Autodesk Inventor part; units mm, degrees
ref_plane "YZ Plane" through (0, 0, 0) normal (1, 0, 0) x (0, 1, 0)
ref_plane "XZ Plane" through (0, 0, 0) normal (0, 1, 0) x (-1, 0, 0)
ref_plane "XY Plane" through (0, 0, 0) normal (0, 0, 1) x (1, 0, 0)
sketch "Sketch1" plane through (0, 0, 0) normal (0, 0, 1) x (1, 0, 0)
  line L0 (-568.325, -1219.2) -> (568.325, -1219.2)
  line L1 (568.325, -1219.2) -> (568.325, 1219.2)
  line L2 (568.325, 1219.2) -> (-568.325, 1219.2)
  line L3 (-568.325, 1219.2) -> (-568.325, -1219.2)
  line L4 (-568.325, -1219.2) -> (568.325, 1219.2) construction
  line L5 (568.325, -1219.2) -> (-568.325, 1219.2) construction
  line L6 (568.325, 1219.2) -> (-568.325, -1219.2)
  line L7 (-528.0371, -1237.98) -> (-608.6129, -1200.42)
  line L8 (608.6129, 1200.42) -> (528.0371, 1237.98)
  line L9 (528.0371, 1237.98) -> (-608.6129, -1200.42)
  line L10 (-528.0371, -1237.98) -> (608.6129, 1200.42)
  point P0 (0, 0)
  point P1 (519.2829, 1219.2)
  point P2 (-568.325, -1113.9923)
  point P3 (-519.2829, -1219.2)
  point P4 (568.325, 1113.9923)
  dimension "d0" = 1136.65
  dimension "d1" = 2438.4
  dimension "d2" = 88.9
  dimension "d3" = 88.9
extrude "Extrusion1" add sketch "Sketch1" along normal blind 38.1 contours L6 L1 L10 L0 | L3 L9 L2 L6
properties part number "S_2x4x105.918"
Input: part model. Units: mm. Frame: model coordinates. Coordinates: 2 decimals unless noted, no trailing zeros. Order: outer loops, then holes, each group sorted by start corner. A loop starts at its lowest first (then second) coordinate and runs counter-clockwise, first axis right, second up. Notation, with made-up numbers: M 49.5,61.25 L 106.5,61.25 A24 ccw 106.5,88.25 Z; hole C 59,-19 d7. An arc over 180 degrees is marked long. Answer as CSV lines item,"result".
1. First-contact query: P1, Ø2, axis at x = 380, z = 18.5, coming from the +Y side; P2, Ø2, axis at x = 186, z = 31.5, coming from the -Y side; P3, Ø3, axis at x = 394.5, z = 20.5, coming from the -Y side. Flat tips, straight axial feed; report the tip coordinate or a pass-through.
Reported:
P1,"y = 922.55"
P2,"y = 291.66"
P3,"y = 737.88"
2. Section A-A (z = 6). Return the cut outline in (x, y) (3 decimals).
Reported:
outline,"M -568.325,-1219.2 L -519.283,-1219.2 L 568.325,1113.992 L 568.325,1219.2 L 519.283,1219.2 L -568.325,-1113.992 Z"
3. Section C-C (x = 348.5). Return the cut outline in (y, z).
Reported:
outline,"M 642.41,0 L 852.83,0 L 852.83,38.1 L 642.41,38.1 Z"
4. Material intervals for line 1 (Y direction, x = -56, z = 34); line 2 (X direction, y = 958.5, z = 34.5); line 3 (X direction, y = 740, z = 33), sorted ascending. Write a range as from..to.
Reported:
line 1,"-225.34..-14.93"
line 2,"397.76..495.84"
line 3,"295.91..393.99"
5. Section B-B (y = -68.5). Return the cut outline in (x, z).
Reported:
outline,"M -80.97,0 L 17.11,0 L 17.11,38.1 L -80.97,38.1 Z"
